Can you work these out from the model? Positions are in its coordinate system, mm. Face numbers are marked on the shaded views. Coordinates: 2 decimals unless noted, no trailing zeros. Order: outer loops, then holes, each group sorted by start corner. A loop starts at its lowest first (then second) coordinate and runs counter-clockwise, first axis right, second up.
```python
from build123d import *

# Parameters (mm, degrees)
CYLINDER003_R     = 0.75
CYLINDER003_DEPTH = 10
ARRAY_COUNT       = 4
CYLINDER002_R     = 4.35
CYLINDER002_DEPTH = 10
CYLINDER001_R     = 10.9
CYLINDER001_DEPTH = 10
TORUS_R           = 1.5
CYLINDER_R        = 28
CYLINDER_DEPTH    = 6


with BuildPart() as array:
    # Cylinder003 → Cylinder003 (new body)
    with BuildSketch(Plane(origin=(7.3, 0, -6), x_dir=(1, 0, 0), z_dir=(0, 0, 1))):
        Circle(CYLINDER003_R)
    extrude(amount=CYLINDER003_DEPTH)

    # Array: Array ×4 about axis
    array_axis = Axis((0, 0, 0), (0, 0, 1))


with BuildPart() as array_1:
    add(array.part)
    for i in range(1, ARRAY_COUNT):
        add(array.part.rotate(array_axis, i * 360 / ARRAY_COUNT))


with BuildPart() as hueco_eje:
    # Cylinder002 → Cylinder002 (new body)
    with BuildSketch(Plane.XY.offset(-6)):
        Circle(CYLINDER002_R)
    extrude(amount=CYLINDER002_DEPTH)


with BuildPart() as corona_servo:
    # Cylinder001 → Cylinder001 (new body)
    with BuildSketch(Plane.XY.offset(1)):
        Circle(CYLINDER001_R)
    extrude(amount=CYLINDER001_DEPTH)


with BuildPart() as obj1:
    # Torus → Torus (revolve)
    with BuildSketch(Plane.XZ):
        with Locations((28, 0)):
            Circle(TORUS_R)
    revolve(axis=Axis((0, 0, 0), (0, 0, 1)))


with BuildPart() as obj2:
    # Cylinder → Cylinder (new body)
    with BuildSketch(Plane.XY.offset(-3)):
        Circle(CYLINDER_R)
    extrude(amount=CYLINDER_DEPTH)

    # Cut: cut obj1
    add(obj1.part, mode=Mode.SUBTRACT)

    # Cut001: cut corona servo
    add(corona_servo.part, mode=Mode.SUBTRACT)

    # Cut002: cut hueco-eje
    add(hueco_eje.part, mode=Mode.SUBTRACT)

    # Cut003: cut Array
    add(array_1.part, mode=Mode.SUBTRACT)


solid = obj2.part
```
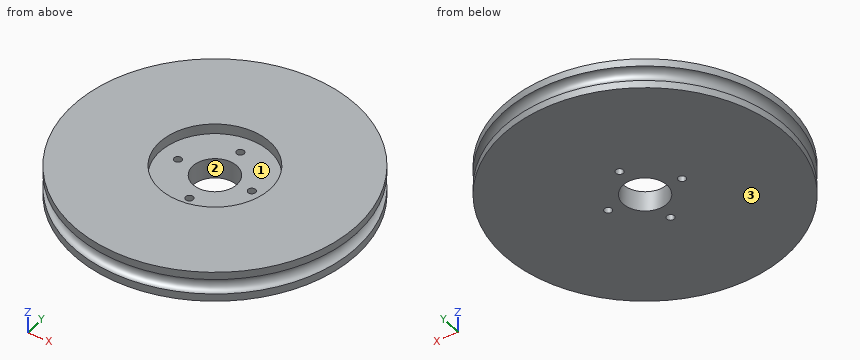
1. Thinking about a two-plate mould opening in Y: for the marked faces 1, 2 and 3, which applies, pulls with the +Y half, pulls with the -Y half, needs draft (parallel to the pull), parting line crosses it, or undercut?
Completed:
face 1: undercut
face 2: undercut
face 3: needs draft
2. Imagine slicing it at C-C on z = -0.3. Please give me the cut outline in (x, y).
Completed:
outline: circle Ø53.06 at (0, 0); hole circle Ø1.5 at (-7.3, 0); hole circle Ø8.7 at (0, 0); hole circle Ø1.5 at (0, -7.3); hole circle Ø1.5 at (0, 7.3); hole circle Ø1.5 at (7.3, 0)
3. I'm going to push flat-ended pins straight in: pin 1 (6.5 mm diameter, centred on x = 2.5, y = 1, fed in from +Z); pin 2 (1.5 mm diameter, centred on y = 11, z = 0, fed in from -X); pin 3 (1.2 mm diameter, centred on x = 7.3, y = 0, fed in from -Z). Where does each tip first touch, or does it pass through?
Completed:
pin 1: stops at z = 1
pin 2: stops at x = -24.45
pin 3: passes through
4. Please list where these lines run through material, in increasing order: probe 1 along Z at (x, y) = (-4.5, -6); probe 2 along Y at (x, z) = (-1, 2.15); probe 3 along X at (y, z) = (7.3, -2).
Completed:
probe 1: z = -3 to 1
probe 2: y = -27.98 to -10.85, 10.85 to 27.98
probe 3: x = -27.03 to -0.75, 0.75 to 27.03
5. Imagine slicing it at A-A on x = 0. Please give me the cut outline in (y, z), then the cut area to 3 significant figures.
Completed:
outline: (-28, -3) - (-8.05, -3) - (-8.05, 1) - (-10.9, 1) - (-10.9, 3) - (-28, 3) - (-28, 1.5) arc R1.5 cw to (-28, -1.5) - close; (-6.55, -3) - (-4.35, -3) - (-4.35, 1) - (-6.55, 1) - close; (4.35, -3) - (6.55, -3) - (6.55, 1) - (4.35, 1) - close; (8.05, -3) - (28, -3) - (28, -1.5) arc R1.5 cw to (28, 1.5) - (28, 3) - (10.9, 3) - (10.9, 1) - (8.05, 1) - close
area: 239 mm2
